Source: CAD feature listing. Evaluate the final solid. Frame: model axes, mm. Face numbers are marked on the shaded views. A direction names the side the tool comes from. Round coordinates to 2 decimals unless told otherwise and drop trailing zeros. Write each loop counter-clockwise with the first axis right and the second up, starting at its lowest first coordinate (ties: lowest second). Pieces come first, ordered by that corner, then holes.
from build123d import *

# Parameters (mm, degrees)
SKETCH_2_R               = 1
CUT_EXTRUDE_1_DEPTH      = 3
PATTERN_CIRCULAR_1_COUNT = 4
SKETCH_5_R               = 1
CUT_EXTRUDE_2_DEPTH      = 10
PATTERN_CIRCULAR_3_COUNT = 4
SKETCH_7_R               = 2
CUT_EXTRUDE_3_DEPTH      = 1
PATTERN_CIRCULAR_4_COUNT = 4


with BuildPart() as part:
    # Sketch 1 → Revolve 1 (revolve)
    with BuildSketch(Plane.XY):
        Polygon((0, 13), (13, 13), (13, 0), (10, 0), (10, 10), (0, 10), align=None)
    revolve(axis=Axis((0, 0, 0), (1, 0, 0)))

    # Sketch 2 → Cut-Extrude 1 (cut)
    with BuildSketch(Plane(origin=(13, 0, 0), x_dir=(0, 0, -1), z_dir=(1, 0, 0))):
        with Locations((0, 6)):
            Circle(SKETCH_2_R)
    cut_extrude_1 = extrude(amount=-CUT_EXTRUDE_1_DEPTH, mode=Mode.SUBTRACT)

    # Pattern Circular 1: Cut-Extrude 1 ×4 about axis
    pattern_circular_1_axis = Axis((0, 0, 0), (1, 0, 0))
    for i in range(1, PATTERN_CIRCULAR_1_COUNT):
        add(cut_extrude_1.rotate(pattern_circular_1_axis, i * 360 / PATTERN_CIRCULAR_1_COUNT), mode=Mode.SUBTRACT)

    # Sketch 5 → Cut-Extrude 2 (cut)
    with BuildSketch(Plane.XY.offset(13)):
        with Locations((3, 0)):
            Circle(SKETCH_5_R)
    cut_extrude_2 = extrude(amount=-CUT_EXTRUDE_2_DEPTH, mode=Mode.SUBTRACT)

    # Pattern Circular 3: Cut-Extrude 2 ×4 about axis
    pattern_circular_3_axis = Axis((10, 0, 0), (-1, 0, 0))
    for i in range(1, PATTERN_CIRCULAR_3_COUNT):
        add(cut_extrude_2.rotate(pattern_circular_3_axis, i * 360 / PATTERN_CIRCULAR_3_COUNT), mode=Mode.SUBTRACT)

    # Sketch 7 → Cut-Extrude 3 (cut)
    with BuildSketch(Plane.XY.offset(13)):
        with Locations((3, 0)):
            Circle(SKETCH_7_R)
    cut_extrude_3 = extrude(amount=-CUT_EXTRUDE_3_DEPTH, mode=Mode.SUBTRACT)

    # Pattern Circular 4: Cut-Extrude 3 ×4 about axis
    pattern_circular_4_axis = Axis((0, 0, 0), (1, 0, 0))
    for i in range(1, PATTERN_CIRCULAR_4_COUNT):
        add(cut_extrude_3.rotate(pattern_circular_4_axis, i * 360 / PATTERN_CIRCULAR_4_COUNT), mode=Mode.SUBTRACT)


solid = part.part
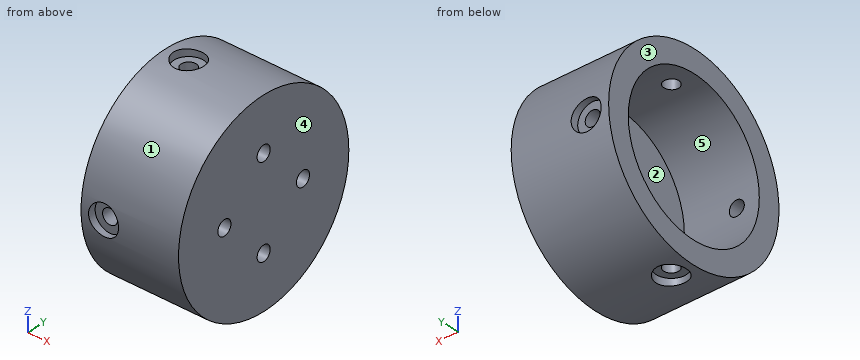
1) Section query A-A on y = 0. State how many separate pieces and enclosed holes the cut face has, then the cut area to 3 significant figures.
Taken from the geometry:
separate pieces: 5
enclosed holes: 0
area: 110 mm2
2) Reachability of the marked faces 4 and 5 from +Z, -Z, +X, -X, +Y, -Y: full face, straight path, thin tool, end or side. Return the list, or none.
Taken from the geometry:
face 4: +Z, -Z, +X, +Y, -Y
face 5: -X
3) Material intervals for line 1 (X direction, y = 0, z = 10.9); line 2 (X direction, y = 1.75, z = -3.25); line 3 (X direction, y = 0, z = -12.25), sorted ascending.
Taken from the geometry:
line 1: x = 0 to 2, 4 to 13
line 2: x = 10 to 13
line 3: x = 0 to 1, 5 to 13
4) Pull-direction query (Z, two-part tool) for the marked faces 1, 2 and 3; classes: released by +Z, released by -Z, zero draft, split by the parting line, or undercut.
Taken from the geometry:
face 1: split by the parting line
face 2: undercut
face 3: zero draft
5) Contact query for flat-ended pins moving along their axis: P1, Ø1.8, axis at x = 3, z = 0, coming from the -Y side; P2, Ø2, axis at x = 3.5, y = 8.5, coming from the +Z side; P3, Ø1.5, axis at x = 2, z = 9, coming from the -Y side; P4, Ø3, axis at x = 3.5, z = -0.5, coming from the -Y side. Output: stop coordinate, or through.
Taken from the geometry:
P1: passes through
P2: stops at z = 10.62
P3: stops at y = -10.05
P4: stops at y = -13
6) Section query D-D on z = 6. Return the cut outline in (x, y).
Taken from the geometry:
outline: (0, -11.53) - (13, -11.53) - (13, -1) - (10, -1) - (10, -8) - (0, -8) - close; (0, 8) - (10, 8) - (10, 1) - (13, 1) - (13, 11.53) - (0, 11.53) - close
